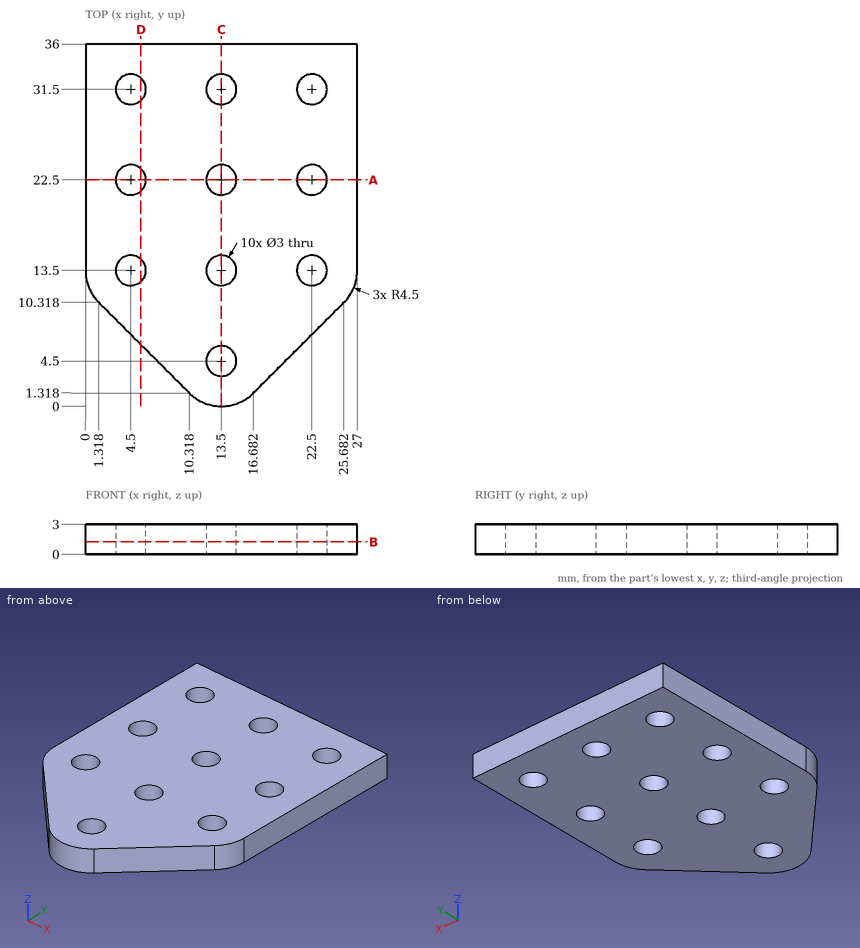
Study the drawing (mm; zero at the part's minimum x, y, z) and answer. Coordinates: 2 decimals unless noted, no trailing zeros. Write each loop counter-clockwise with the first axis right and the second up, starting at its lowest first coordinate (ties: lowest second). Pieces come first, ordered by that corner, then holes. Notation, with made-up numbers: M 23.25,8 L 69.25,8 A19 cw 69.25,26 Z; hole C 33.5,-10.75 d9. An arc over 180 degrees is marked long. Use a Markdown table: item, result. Add a question column.
1. Section A-A (y = 22.5) is taken. Give the vertices of the cut face in (x, z), plus the area to 3 significant figures.
2. Section B-B (z = 1.25) is taken. Count the separate pieces of the cut face and the enclosed holes in it, plus the area to 3 significant figures.
3. Straight lines are drawn through the part: line 1 along Y through (x, z) = (13.5, 1.8); line 2 along X through (y, z) = (13.5, 0.9); line 3 along Y through (x, z) = (4, 1.25). For each, find the intervals that lie inside material, in ascending order. Write a range as [from, to].
4. Given P1, Ø1, axis at y = 6, z = 0.5, coming from the +X side; P2, Ø2.5, axis at x = 4.5, y = 22.5, coming from the +Z side, each flat-ended and moving along its own axis, determine where each tip first touches the part or whether it passes through.
5. Section D-D (x = 5.5) is taken. Give the vertices of the cut face in (y, z), plus the area to 3 significant figures.
6. Section C-C (x = 13.5) is taken. Give the vertices of the cut face in (y, z).
Data:
| question | item | result |
|---|---|---|
| 1 | outline | M 0,0 L 3,0 L 3,3 L 0,3 Z; M 6,0 L 12,0 L 12,3 L 6,3 Z; M 15,0 L 21,0 L 21,3 L 15,3 Z; M 24,0 L 27,0 L 27,3 L 24,3 Z |
| 1 | area | 54.0 mm2 |
| 2 | separate pieces | 1 |
| 2 | enclosed holes | 10 |
| 2 | area | 764 mm2 |
| 3 | line 1 | y = [0, 3], [6, 12], [15, 21], [24, 30], [33, 36] |
| 3 | line 2 | x = [0, 3], [6, 12], [15, 21], [24, 27] |
| 3 | line 3 | y = [7.64, 12.09], [14.91, 21.09], [23.91, 30.09], [32.91, 36] |
| 4 | P1 | stops at x = 21.86 |
| 4 | P2 | passes through |
| 5 | outline | M 6.14,0 L 12.38,0 L 12.38,3 L 6.14,3 Z; M 14.62,0 L 21.38,0 L 21.38,3 L 14.62,3 Z; M 23.62,0 L 30.38,0 L 30.38,3 L 23.62,3 Z; M 32.62,0 L 36,0 L 36,3 L 32.62,3 Z |
| 5 | area | 69.5 mm2 |
| 6 | outline | M 0,0 L 3,0 L 3,3 L 0,3 Z; M 6,0 L 12,0 L 12,3 L 6,3 Z; M 15,0 L 21,0 L 21,3 L 15,3 Z; M 24,0 L 30,0 L 30,3 L 24,3 Z; M 33,0 L 36,0 L 36,3 L 33,3 Z |
